Work out the finished part from the listing and answer in its coordinate system (mm). Face numbers are marked on the shaded views. A direction names the side the tool comes from. Give positions to 0.01 mm unless a question says otherwise; leave off trailing zeros. Order: outer loops, then holes, each group sorted by start corner. A loop starts at its lowest first (then second) coordinate and runs counter-clockwise, first axis right, second up. Notation, with made-up numbers: (64.5, -16) - (117.5, -16) arc R10 ccw to (117.5, -12) - close; hole circle Ø5 at (36.5, -20.75). An arc over 180 degrees is marked (long way). Return JSON: item names as keys, results as strings. Group by question number.
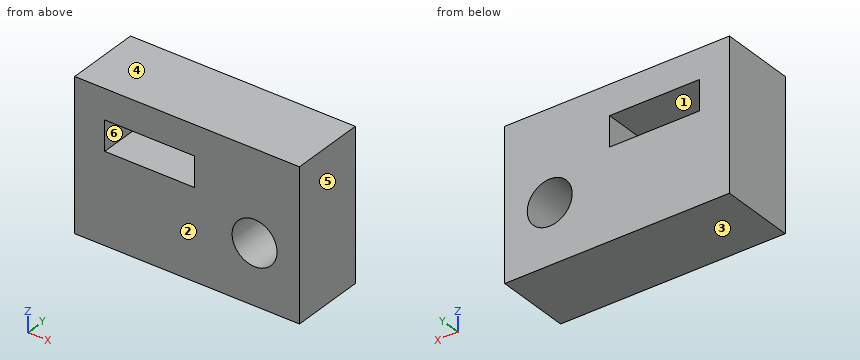
from build123d import *

# Parameters (mm, degrees)
F0_W     = 75
F0_H     = 50
F0_R     = 7.5
F0_W_2   = 30
F0_H_2   = 10
F1_DEPTH = 25


with BuildPart() as f1:
    # F0 (on Front) → F1 (new body)
    with BuildSketch(Plane.XZ):
        with Locations((-22.5, 5)):
            Rectangle(F0_W, F0_H)
        Circle(F0_R, mode=Mode.SUBTRACT)
        with Locations((-35, 15)):
            Rectangle(F0_W_2, F0_H_2, mode=Mode.SUBTRACT)
    extrude(amount=F1_DEPTH)


solid = f1.part
1. The part is cut by section B-B (y = -16.75). Give the vertices of the cut face in (x, z), and give its area (3 significant figures).
2. Determine the mould class of the marked faces 1, 2, 3 and 4 for opening direction Z: released by +Z, released by -Z, zero draft, split by the parting line, or undercut.
3. This flat-tipped pin is pushed along its axis until it touches: pin 1 (9 mm diameter, centred on x = 0, z = 0, fed in from +Y). Where does it stop, or does it pass through?
4. The part is cut by section A-A (x = 0). Give the vertices of the cut face in (y, z), and give its area (3 significant figures).
5. The part is cut by section C-C (z = 0). Give the vertices of the cut face in (x, y).
6. A tool of negligible diameter and unlimited length cuts with its end or side. For the marked faces 5 and 6, from which of +Z, -Z, +X, -X, +Y, -Y can it reach the whole face along a straight path? Write none if from no direction.
7. Consider probe 1 along X at (y, z) = (-17.5, 12); probe 2 along Z at (x, y) = (-38, -23.75); probe 3 along Z at (x, y) = (0, -16.25). Determine where each line is inside the solid, lowest interval first. Write a range as from..to.
Answers:
{
 "1": {"outline": "(-60, -20) - (15, -20) - (15, 30) - (-60, 30) - close; hole (-50, 10) - (-20, 10) - (-20, 20) - (-50, 20) - close; hole circle Ø15 at (0, 0)", "area": "3,270 mm^2"},
 "2": {"face 1": "undercut", "face 2": "zero draft", "face 3": "released by -Z", "face 4": "released by +Z"},
 "3": {"pin 1": "passes through"},
 "4": {"outline": "(-25, -20) - (0, -20) - (0, -7.5) - (-25, -7.5) - close; (-25, 7.5) - (0, 7.5) - (0, 30) - (-25, 30) - close", "area": "875 mm^2"},
 "5": {"outline": "(-60, -25) - (-7.5, -25) - (-7.5, 0) - (-60, 0) - close; (7.5, -25) - (15, -25) - (15, 0) - (7.5, 0) - close"},
 "6": {"face 5": "+Z, -Z, +X, +Y, -Y", "face 6": "+Y, -Y"},
 "7": {"probe 1": "x = -60..-50, -20..15", "probe 2": "z = -20..10, 20..30", "probe 3": "z = -20..-7.5, 7.5..30"}
}
